Autodesk Fusion 360 part; units mm, degrees
sketch "Skizze1" plane through (0, 0, 0) normal (0, 0, 1) x (1, 0, 0)
  line L0 (0, 0) -> (20, 0)
  line L1 (20, 0) -> (20, 20)
  line L2 (20, 20) -> (0, 20)
  line L3 (0, 20) -> (0, 0)
  dimension "d1" = 20
  dimension "d2" = 20
extrude "Extrusion1" add sketch "Skizze1" along normal blind 1.4
sketch "Skizze2" plane through (0, 0, 1.4) normal (0, 0, 1) x (-1, 0, 0)
  line L0 (0, -20) -> (0, 0)
  line L1 (0, 0) -> (-20, 0)
  line L2 (-20, 0) -> (-20, -20)
  line L3 (-20, -20) -> (0, -20)
  line L4 (-15, -15) -> (-5, -15)
  line L5 (-5, -15) -> (-5, -5)
  line L6 (-5, -5) -> (-15, -5)
  line L7 (-15, -5) -> (-15, -15)
  line L8 (-15, -15) -> (-5, -5) construction
  line L9 (-5, -15) -> (-15, -5) construction
  point P0 (-10, -10)
extrude "Extrusion2" add sketch "Skizze2" along normal blind 5 contours L4 L5 L6 L7
chamfer "Fase1" distance 5 angle 45 4 edges at (10, 5, 1.4) (5, 10, 1.4) (10, 15, 1.4) (15, 10, 1.4)
sketch "Skizze3" plane through (0, 0, 0) normal (0, 1, 0) x (1, 0, 0)
  line L0 (0, 0) -> (0, -1.4)
  line L1 (0, -1.4) -> (20, -1.4)
  line L2 (10, -1.4) -> (10, -4.4)
  line L3 (10, -4.4) -> (7, -4.4)
  line L4 (7, -4.4) -> (13, -4.4)
  line L5 (13, -4.4) -> (13, -1.4)
  line L6 (13, -1.4) -> (7, -1.4)
  line L7 (7, -1.4) -> (7, -4.4)
  line L8 (7, -4.4) -> (5, -4.4)
  line L9 (5, -4.4) -> (15, -4.4)
  line L10 (15, -4.4) -> (15, -1.4)
  line L11 (15, -1.4) -> (5, -1.4)
  line L12 (5, -1.4) -> (5, -4.4)
  dimension "d8" = 2
extrude "Extrusion3" cut sketch "Skizze3" along normal blind 21
sketch "Skizze4" plane through (0, 0, 0) normal (1, 0, 0) x (0, 1, 0)
  line L0 (0, 0) -> (0, 1.4)
  line L1 (0, 1.4) -> (5, 1.4)
  line L2 (5, 1.4) -> (15, 1.4)
  line L3 (15, 1.4) -> (15, 4.4)
  line L4 (15, 4.4) -> (5, 4.4)
  line L5 (5, 4.4) -> (5, 1.4)
  dimension "d11" = 10
  dimension "d12" = 3
Geometry: final body of the model. Coordinates: model frame, mm. A direction names the side the tool comes from. Coordinates: 2 decimals unless noted, no trailing zeros. Loops run counter-clockwise (first coordinate to the right, second up) from the corner with the lowest first, then second, coordinate; pieces in that order, holes last. Notation, with made-up numbers: M 26,50 L 83,50 A11 cw 83,63 Z; hole C 70,53 d2. An arc over 180 degrees is marked long. Put each result on its own line as item: value.
(1) Material intervals for probe 1 along Z at (x, y) = (10, 8.75); probe 2 along Z at (x, y) = (5.5, 16); probe 3 along X at (y, z) = (11.5, 2.5), sorted ascending.
Answer sheet:
probe 1: z = 0 to 1.4, 4.4 to 6.4
probe 2: z = 0 to 1.4, 4.4 to 5.4
probe 3: x = 1.1 to 5, 15 to 18.9
(2) First-contact query: pin 1 (2 mm diameter, centred on x = 17.5, z = 2.5, fed in from +Y); pin 2 (1 mm diameter, centred on x = 2, y = 10.5, fed in from +Z); pin 3 (1 mm diameter, centred on x = 8, y = 4, fed in from +Z). Flat tips, straight axial feed; report the tip coordinate or a pass-through.
Answer sheet:
pin 1: stops at y = 19.9
pin 2: stops at z = 3.9
pin 3: stops at z = 5.9
(3) Access query for faces 5 (the face through (15, 10, 3)), 6 (the face through (10, 20, 1)). Directions: +Z, -Z, +X, -X, +Y, -Y. A direction counts if a zero-diameter tool reaches every point of the face in a straight line with its end or side. Return the directions, or none.
Answer sheet:
face 5: +Y, -Y
face 6: +Z, -Z, +X, -X, +Y
(4) Cut plane C-C on z = 3.25. Return the cut outline in (x, y).
Answer sheet:
outline: M 1.85,1.85 L 5,1.85 L 5,18.15 L 1.85,18.15 Z; M 15,1.85 L 18.15,1.85 L 18.15,18.15 L 15,18.15 Z
(5) Draft query along X for faces 1 (the face through (18, 9.9, 3.4)), 2 (the face through (10, 10, 1.4)), 3 (the face through (0, 10, 1)), 4 (the face through (5, 10, 3)). Return one class per face: pulls with the +X half, pulls with the -X half, needs draft (parallel to the pull), parting line crosses it, or undercut.
Answer sheet:
face 1: pulls with the +X half
face 2: undercut
face 3: pulls with the -X half
face 4: undercut
